Read the model definition and answer for the solid it produces. Units are mm, in the model's axes. Coordinates: 2 decimals unless noted, no trailing zeros. Write each loop counter-clockwise with the first axis right and the second up, starting at its lowest first coordinate (ties: lowest second). Pieces come first, ordered by that corner, then holes.
1) Each of these flat-tipped pins is pushed along its axis until it touches: pin 1 Ø0.8 at (y, z) = (-2, -4) entering from +X; pin 2 Ø0.6 at (y, z) = (-1.5, 3.5) entering from -X. Where does it stop, or does it pass through?
2) The part is cut by section A-A (x = -4.25). Determine the outline of the cut face in (y, z).
3) Find the intervals of material crossed by line 1 (Y direction, x = 10.75, z = -3.25); line 2 (Z direction, x = 4.25, y = -2.5); line 3 (X direction, y = 6.75, z = -6), in increasing order.
4) The part is cut by section B-B (z = 0). Determine the outline of the cut face in (x, y).
from build123d import *

# Parameters (mm, degrees)
SKETCH_1_W      = 29
SKETCH_1_H      = 12.7
EXTRUDE_1_DEPTH = 15.7
EXTRUDE_2_DEPTH = 3.5
FILLET_1_R      = 0.05
CHAMFER_1_SIZE  = 1.5
FILLET_2_R      = 0.75


with BuildPart() as part:
    # Эскиз1 → Бобышка-Вытянуть1 (new body)
    with BuildSketch(Plane(origin=(0, 0, 0), x_dir=(1, 0, 0), z_dir=(0, 1, 0))):
        Rectangle(SKETCH_1_W, SKETCH_1_H)
    extrude(amount=EXTRUDE_1_DEPTH)

    # Эскиз2 → Бобышка-Вытянуть2 (add)
    with BuildSketch(Plane.XZ):
        with BuildLine():
            Line((-12.3, 4.15), (-11.9, 4.15))
            ThreePointArc((-11.9, 4.15), (-11.864644661, 4.135355339), (-11.85, 4.1))
            Line((-11.85, 4.1), (-11.85, 3.4))
            ThreePointArc((-11.85, 3.4), (-11.864644661, 3.364644661), (-11.9, 3.35))
            Line((-11.9, 3.35), (-12.3, 3.35))
            ThreePointArc((-12.3, 3.35), (-12.335355339, 3.364644661), (-12.35, 3.4))
            Line((-12.35, 3.4), (-12.35, 4.1))
            ThreePointArc((-12.35, 4.1), (-12.335355339, 4.135355339), (-12.3, 4.15))
        make_face()
        with BuildLine():
            Line((7.65, -3.4), (7.65, -4.1))
            ThreePointArc((7.65, -4.1), (7.664644661, -4.135355339), (7.7, -4.15))
            Line((7.7, -4.15), (8.1, -4.15))
            ThreePointArc((8.1, -4.15), (8.135355339, -4.135355339), (8.15, -4.1))
            Line((8.15, -4.1), (8.15, -3.4))
            ThreePointArc((8.15, -3.4), (8.135355339, -3.364644661), (8.1, -3.35))
            Line((8.1, -3.35), (7.7, -3.35))
            ThreePointArc((7.7, -3.35), (7.664644661, -3.364644661), (7.65, -3.4))
        make_face()
        with BuildLine():
            Line((-12.35, -3.4), (-12.35, -4.1))
            ThreePointArc((-12.35, -4.1), (-12.335355339, -4.135355339), (-12.3, -4.15))
            Line((-12.3, -4.15), (-11.9, -4.15))
            ThreePointArc((-11.9, -4.15), (-11.864644661, -4.135355339), (-11.85, -4.1))
            Line((-11.85, -4.1), (-11.85, -3.4))
            ThreePointArc((-11.85, -3.4), (-11.864644661, -3.364644661), (-11.9, -3.35))
            Line((-11.9, -3.35), (-12.3, -3.35))
            ThreePointArc((-12.3, -3.35), (-12.335355339, -3.364644661), (-12.35, -3.4))
        make_face()
        with BuildLine():
            Line((11.2, 4.15), (11.6, 4.15))
            ThreePointArc((11.6, 4.15), (11.635355339, 4.135355339), (11.65, 4.1))
            Line((11.65, 4.1), (11.65, 3.4))
            ThreePointArc((11.65, 3.4), (11.635355339, 3.364644661), (11.6, 3.35))
            Line((11.6, 3.35), (11.2, 3.35))
            ThreePointArc((11.2, 3.35), (11.164644661, 3.364644661), (11.15, 3.4))
            Line((11.15, 3.4), (11.15, 4.1))
            ThreePointArc((11.15, 4.1), (11.164644661, 4.135355339), (11.2, 4.15))
        make_face()
        with BuildLine():
            Line((4.2, 4.15), (4.6, 4.15))
            ThreePointArc((4.6, 4.15), (4.635355339, 4.135355339), (4.65, 4.1))
            Line((4.65, 4.1), (4.65, 3.4))
            ThreePointArc((4.65, 3.4), (4.635355339, 3.364644661), (4.6, 3.35))
            Line((4.6, 3.35), (4.2, 3.35))
            ThreePointArc((4.2, 3.35), (4.164644661, 3.364644661), (4.15, 3.4))
            Line((4.15, 3.4), (4.15, 4.1))
            ThreePointArc((4.15, 4.1), (4.164644661, 4.135355339), (4.2, 4.15))
        make_face()
    extrude(amount=EXTRUDE_2_DEPTH)

    # Скругление1
    fillet_1_edges = [part.edges().sort_by_distance(p)[0] for p in [
        (-12.335355339, -3.5, -4.135355339),
        (-12.1, -3.5, -4.15),
        (-11.864644661, -3.5, -4.135355339),
        (-11.85, -3.5, -3.75),
        (-11.864644661, -3.5, -3.364644661),
        (-12.1, -3.5, -3.35),
        (-12.335355339, -3.5, -3.364644661),
        (-12.35, -3.5, -3.75),
        (-12.335355339, -3.5, 3.364644661),
        (-12.1, -3.5, 3.35),
        (-11.864644661, -3.5, 3.364644661),
        (-11.85, -3.5, 3.75),
        (-11.864644661, -3.5, 4.135355339),
        (-12.1, -3.5, 4.15),
        (-12.335355339, -3.5, 4.135355339),
        (-12.35, -3.5, 3.75),
        (7.664644661, -3.5, -4.135355339),
        (7.9, -3.5, -4.15),
        (8.135355339, -3.5, -4.135355339),
        (8.15, -3.5, -3.75),
        (8.135355339, -3.5, -3.364644661),
        (7.9, -3.5, -3.35),
        (7.664644661, -3.5, -3.364644661),
        (7.65, -3.5, -3.75),
    ]]
    fillet(fillet_1_edges, radius=FILLET_1_R)

    # Фаска1
    chamfer_1_edges = [part.edges().sort_by_distance(p)[0] for p in [
        (14.5, 15.7, 0),
    ]]
    chamfer(chamfer_1_edges, length=CHAMFER_1_SIZE)

    # Скругление2
    fillet_2_edges = [part.edges().sort_by_distance(p)[0] for p in [
        (-14.5, 15.7, 0),
        (-0.75, 15.7, 6.35),
        (-0.75, 15.7, -6.35),
        (13, 15.7, 0),
        (14.5, 7.1, -6.35),
        (13.75, 14.95, -6.35),
        (14.5, 7.1, 6.35),
        (14.5, 14.2, 0),
        (13.75, 14.95, 6.35),
        (-14.5, 7.85, 6.35),
        (-14.5, 7.85, -6.35),
    ]]
    fillet(fillet_2_edges, radius=FILLET_2_R)


solid = part.part
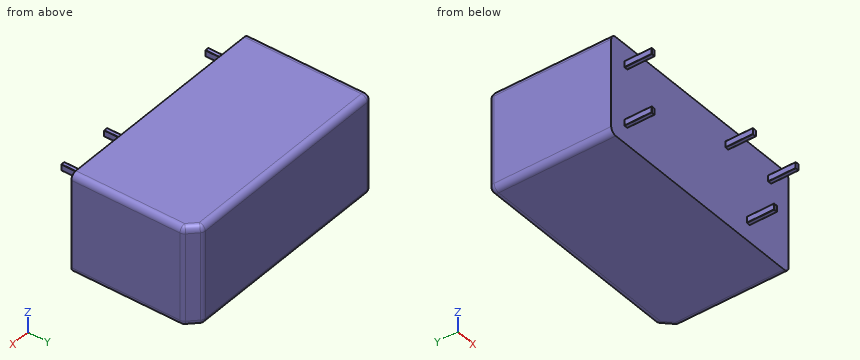
Reported:
1. pin 1: stops at x = 8.15
1. pin 2: stops at x = -12.35
2. outline: (0, -6.35) - (14.95, -6.35) arc R0.75 ccw to (15.7, -5.6) - (15.7, 5.6) arc R0.75 ccw to (14.95, 6.35) - (0, 6.35) - close
3. line 1: y = 0 to 15.7
3. line 2: z = 3.35 to 4.15
3. line 3: x = -14.38 to 14.38
4. outline: (-14.5, 0) - (14.5, 0) - (14.5, 13.89) arc R0.75 ccw to (14.28, 14.42) - (13.22, 15.48) arc R0.75 ccw to (12.69, 15.7) - (-13.75, 15.7) arc R0.75 ccw to (-14.5, 14.95) - close
